Could you check a few things on this drawing? It's one solid part, dimensions in mm from its lowest x, y, z. Give positions to 0.01 mm unless a question says otherwise; leave off trailing zeros. Loops run counter-clockwise (first coordinate to the right, second up) from the corner with the lowest first, then second, coordinate; pieces in that order, holes last. Notation, with made-up numbers: (-0.75, -35) - (48.25, -35) arc R24 cw to (48.25, -2) - close; hole circle Ø11 at (-28, -2). An arc over 180 degrees is marked (long way). Return JSON: item names as keys, results as strings. Group by question number.
(1) If we section it at A-A (y = 35.5): Please give me the cut outline in (x, z), then the cut area to 3 significant figures.
(2) For P1, Ø1.8, axis at x = 38, y = 35.5, coming from the -Z side, with a flat end and sliding along its axis, tell me the tip position at first contact or that it passes through.
(3) I need wall thicknesses on probe 1 along Y at (x, z) = (8, 1.7); probe 2 along Y at (x, z) = (22, 1.05); probe 3 along X at (y, z) = (5, 0.85). Which ranges of each line are inside material? Lowest first, please. Write a range as [from, to].
(4) If we section it at C-C (z = 2.6): Please give me the cut outline in (x, y), then the cut area to 3 significant figures.
(5) If we section it at B-B (y = 20): Please give me the cut outline in (x, z).
(6) If we section it at D-D (x = 22.5): Please give me the cut outline in (y, z).
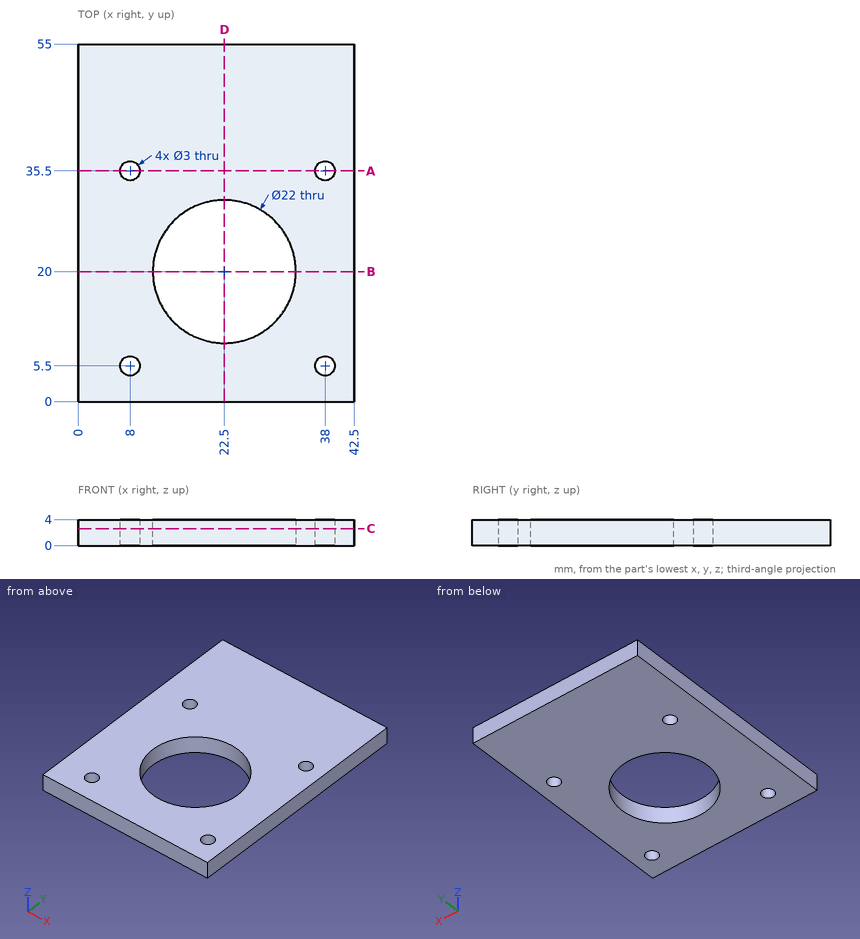
Values:
{
 "1": {"outline": "(0, 0) - (6.5, 0) - (6.5, 4) - (0, 4) - close; (9.5, 0) - (36.5, 0) - (36.5, 4) - (9.5, 4) - close; (39.5, 0) - (42.5, 0) - (42.5, 4) - (39.5, 4) - close", "area": "146 mm2"},
 "2": {"P1": "through"},
 "3": {"probe 1": "[0, 4], [7, 34], [37, 55]", "probe 2": "[0, 9.01], [30.99, 55]", "probe 3": "[0, 6.59], [9.41, 36.59], [39.41, 42.5]"},
 "4": {"outline": "(0, 0) - (42.5, 0) - (42.5, 55) - (0, 55) - close; hole circle Ø3 at (8, 5.5); hole circle Ø3 at (8, 35.5); hole circle Ø22 at (22.5, 20); hole circle Ø3 at (38, 5.5); hole circle Ø3 at (38, 35.5)", "area": "1,930 mm2"},
 "5": {"outline": "(0, 0) - (11.5, 0) - (11.5, 4) - (0, 4) - close; (33.5, 0) - (42.5, 0) - (42.5, 4) - (33.5, 4) - close"},
 "6": {"outline": "(0, 0) - (9, 0) - (9, 4) - (0, 4) - close; (31, 0) - (55, 0) - (55, 4) - (31, 4) - close"}
}
